Can you work these out from the model? Positions are in its coordinate system, mm. Round coordinates to 2 decimals unless told otherwise and drop trailing zeros. Loops run counter-clockwise (first coordinate to the right, second up) from the corner with the lowest first, then second, coordinate; pieces in that order, holes last. Notation, with made-up numbers: (89, 26) -> (118, 26) arc R25 cw to (118, 50) -> close; hole circle Ø5 at (16.5, 74). An arc over 180 degrees is marked (long way). Answer as a JSON object with one key per item and string values.
```python
from build123d import *

# Parameters (mm, degrees)
SKETCH1_R           = 2.4892
BOSS_EXTRUDE1_DEPTH = 6.35
FILLET1_R           = 6.35


with BuildPart() as part:
    # Sketch1 → Boss-Extrude1 (new body)
    with BuildSketch(Plane.XY):
        Polygon((0, 0), (25.4, 0), (101.6, 25.4), (101.6, 76.2), (25.4, 101.6), (0, 101.6), align=None)
        with Locations((36.195, 63.5)):
            Circle(SKETCH1_R, mode=Mode.SUBTRACT)
        with Locations((86.995, 63.5)):
            Circle(SKETCH1_R, mode=Mode.SUBTRACT)
        with Locations((86.995, 50.8)):
            Circle(SKETCH1_R, mode=Mode.SUBTRACT)
        with Locations((86.995, 38.1)):
            Circle(SKETCH1_R, mode=Mode.SUBTRACT)
        with Locations((36.195, 50.8)):
            Circle(SKETCH1_R, mode=Mode.SUBTRACT)
        with Locations((36.195, 38.1)):
            Circle(SKETCH1_R, mode=Mode.SUBTRACT)
        with Locations((12.7, 88.9)):
            Circle(SKETCH1_R, mode=Mode.SUBTRACT)
        with Locations((12.7, 63.5)):
            Circle(SKETCH1_R, mode=Mode.SUBTRACT)
        with Locations((12.7, 38.1)):
            Circle(SKETCH1_R, mode=Mode.SUBTRACT)
        with Locations((12.7, 12.7)):
            Circle(SKETCH1_R, mode=Mode.SUBTRACT)
    extrude(amount=BOSS_EXTRUDE1_DEPTH)

    # Fillet1
    fillet1_edges = [part.edges().sort_by_distance(p)[0] for p in [
        (0, 0, 3.175),
        (25.4, 0, 3.175),
        (101.6, 25.4, 3.175),
        (101.6, 76.2, 3.175),
        (25.4, 101.6, 3.175),
        (0, 101.6, 3.175),
    ]]
    fillet(fillet1_edges, radius=FILLET1_R)


solid = part.part
```
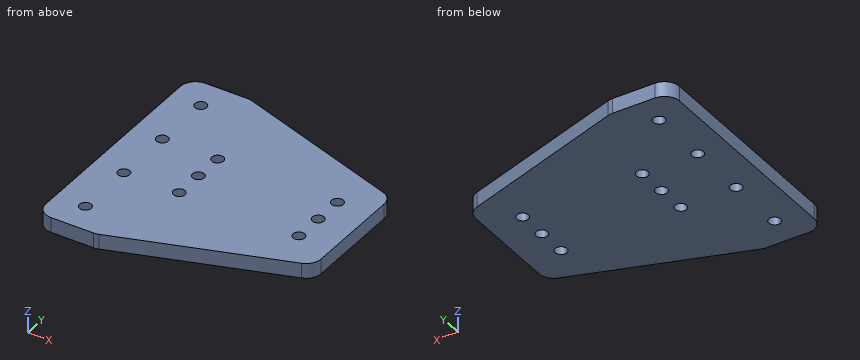
Q1. I want a section at A-A, the plane x = 12.7. Write out the boundary of the cut face in (y, z), then the cut area to 3 significant figures.
Determined:
{"outline": "(0, 0) -> (10.21, 0) -> (10.21, 6.35) -> (0, 6.35) -> close; (15.19, 0) -> (35.61, 0) -> (35.61, 6.35) -> (15.19, 6.35) -> close; (40.59, 0) -> (61.01, 0) -> (61.01, 6.35) -> (40.59, 6.35) -> close; (65.99, 0) -> (86.41, 0) -> (86.41, 6.35) -> (65.99, 6.35) -> close; (91.39, 0) -> (101.6, 0) -> (101.6, 6.35) -> (91.39, 6.35) -> close", "area": "519 mm²"}
Q2. I want a section at D-D, the plane y = 88.9. Write out the boundary of the cut face in (x, z).
Determined:
{"outline": "(0, 0) -> (10.21, 0) -> (10.21, 6.35) -> (0, 6.35) -> close; (15.19, 0) -> (63.5, 0) -> (63.5, 6.35) -> (15.19, 6.35) -> close"}
Q3. I want a section at B-B, the plane y = 63.5. Write out the boundary of the cut face in (x, z).
Determined:
{"outline": "(0, 0) -> (10.21, 0) -> (10.21, 6.35) -> (0, 6.35) -> close; (15.19, 0) -> (33.71, 0) -> (33.71, 6.35) -> (15.19, 6.35) -> close; (38.68, 0) -> (84.51, 0) -> (84.51, 6.35) -> (38.68, 6.35) -> close; (89.48, 0) -> (101.6, 0) -> (101.6, 6.35) -> (89.48, 6.35) -> close"}
Q4. If I drill on L1, parallel to Y at x = 12.7, z = 3.25; L2, parallel to X at y = 64.5, z = 1; L3, parallel to Y at x = 92, z = 4.75, over which ranges is the centre line in solid material (lowest first)? Write a range as [from, to].
Determined:
{"L1": "[0, 10.21], [15.19, 35.61], [40.59, 61.01], [65.99, 86.41], [91.39, 101.6]", "L2": "[0, 10.42], [14.98, 33.92], [38.47, 84.72], [89.27, 101.6]", "L3": "[22.2, 79.4]"}
Q5. I want a section at C-C, the plane z = 4.75. Give the number of separate pieces and of enclosed holes in the cut face, then the cut area to 3 significant figures.
Determined:
{"separate pieces": "1", "enclosed holes": "10", "area": "8,170 mm²"}
Q6. I'm going to push flat-ended pins straight in: pin 1 (1 mm diameter, centred on x = 49, z = 1, fed in from -Y); pin 2 (1.5 mm diameter, centred on x = 45, z = 2, fed in from -Y); pin 3 (4.5 mm diameter, centred on x = 12.7, y = 88.9, fed in from -Z). Where does each tip first touch, or does it pass through?
Determined:
{"pin 1": "y = 7.7", "pin 2": "y = 6.28", "pin 3": "through"}
